Source: CAD feature listing. Evaluate the final solid. Frame: model axes, mm. A direction names the side the tool comes from. Coordinates: 2 decimals unless noted, no trailing zeros. Write each loop counter-clockwise with the first axis right and the second up, starting at its lowest first coordinate (ties: lowest second). Pieces come first, ordered by that corner, then holes. Notation, with made-up numbers: M -27,87 L 13,87 A24 cw 13,125 Z; hole C 85.5,-34 d11. An arc over 180 degrees is marked long. Answer as CSV lines item,"result". Start each with the question number.
1. Section A-A on y = 56.35. Return the cut outline in (x, z) (3 decimals), plus the area to 3 significant figures.
2. Section B-B on z = 1.75. Count the separate pieces of the cut face and the enclosed holes in it, plus the area to 3 significant figures.
3. Section D-D on y = 0. Return the cut outline in (x, z) (3 decimals).
4. Mould query, pull axis Y, two halves, no side actions, for faces 1 (the face through (0, 62.7, 2)), 2 (the face through (-50, 28, 2)), 3 (the face through (-42, 5, 3.175)). Classes: pulls with the +Y half, pulls with the -Y half, needs draft (parallel to the pull), parting line crosses it, or undercut.
5. Contact query for flat-ended pins moving along their axis: pin 1 Ø1.6 at (x, z) = (-58, 2) entering from +Y; pin 2 Ø2 at (x, z) = (48.5, 0.5) entering from -Y; pin 3 Ø3 at (x, z) = (-18.5, 3.5) entering from +Y; pin 4 Ø1.5 at (x, z) = (6, 4) entering from +Y. Output: stop coordinate, or through.
6. Reachability of faces 4 (the face through (-56, 6.35, 2)), 5 (the face through (6.35, 56, 2)), 6 (the face through (1, -40, 2)), 7 (the face through (-6.35, -56, 2)) from +Z, -Z, +X, -X, +Y, -Y: full face, straight path, thin tool, end or side. Return the list, or none.
7. Line query: probe 1 along Y at (x, z) = (43.5, 0.25); probe 2 along Y at (x, z) = (0, 1.9); probe 3 along X at (y, z) = (31, 1.45). Output: solid intervals per line, ascending. Write a range as [from, to].
Autodesk Fusion 360 part; units mm, degrees
sketch "Sketch1" plane through (0, 0, 0) normal (0, 0, 1) x (1, 0, 0) in component "Bracket"
  line L0 (-40, 40) -> (40, 40)
  line L1 (40, 40) -> (40, -40)
  line L2 (40, -40) -> (-40, -40)
  line L3 (-40, -40) -> (-40, 40)
  line L4 (-50, 50) -> (50, 50)
  line L5 (50, 50) -> (50, -50)
  line L6 (50, -50) -> (-50, -50)
  line L7 (-50, -50) -> (-50, 50)
  circle A0 centre (-43.75, 43.75) radius 1
  circle A1 centre (-43.75, -43.75) radius 1
  circle A2 centre (43.75, -43.75) radius 1
  circle A3 centre (43.75, 43.75) radius 1
  line L8 (-6.35, 50) -> (-6.35, 62.7)
  line L9 (-6.35, 62.7) -> (6.35, 62.7)
  line L10 (6.35, 62.7) -> (6.35, 50)
  line L11 (-50, 6.35) -> (-62.7, 6.35)
  line L12 (-62.7, 6.35) -> (-62.7, -6.35)
  line L13 (-62.7, -6.35) -> (-50, -6.35)
  line L14 (-6.35, -50) -> (-6.35, -62.7)
  line L15 (-6.35, -62.7) -> (6.35, -62.7)
  line L16 (6.35, -62.7) -> (6.35, -50)
  line L17 (50, 6.35) -> (62.7, 6.35)
  line L18 (62.7, 6.35) -> (62.7, -6.35)
  line L19 (62.7, -6.35) -> (50, -6.35)
  circle A4 centre (56.35, 0) radius 2.5
  circle A5 centre (0, 56.35) radius 2.5
  circle A6 centre (-56.35, 0) radius 2.5
  circle A7 centre (0, -56.35) radius 2.5
  circle A8 centre (43.75, 43.75) radius 4
  circle A9 centre (-43.75, 43.75) radius 4
  circle A10 centre (-43.75, -43.75) radius 4
  circle A11 centre (43.75, -43.75) radius 4
  dimension "d1" = 80
  dimension "d2" = 80
  dimension "d3" = 100
  dimension "d4" = 100
  dimension "d5" = 40
  dimension "d6" = 50
  dimension "d7" = 40
  dimension "d8" = 50
  dimension "d11" = 2
  dimension "d12" = 2
  dimension "d13" = 2
  dimension "d14" = 2
  dimension "d15" = 87.5
  dimension "d16" = 87.5
  dimension "d17" = 43.75
  dimension "d18" = 43.75
  dimension "d19" = 12.7
  dimension "d20" = 12.7
  dimension "d21" = 6.35
  dimension "d22" = 12.7
  dimension "d23" = 12.7
  dimension "d24" = 6.35
  dimension "d25" = 12.7
  dimension "d26" = 12.7
  dimension "d27" = 6.35
  dimension "d28" = 12.7
  dimension "d29" = 12.7
  dimension "d30" = 6.35
  dimension "d31" = 5
  dimension "d32" = 6.35
  dimension "d33" = 6.35
  dimension "d34" = 5
  dimension "d35" = 6.35
  dimension "d36" = 6.35
  dimension "d37" = 5
  dimension "d38" = 6.35
  dimension "d39" = 6.35
  dimension "d40" = 5
  dimension "d41" = 6.35
  dimension "d42" = 6.35
  dimension "d43" = 8
  dimension "d44" = 8
  dimension "d45" = 8
  dimension "d46" = 8
extrude "Extrude1" add sketch "Sketch1" along normal blind 3.175 contours L4 L5 L6 L7 | L4 L8 L9 L10 | L7 L11 L12 L13 | L5 L17 L18 L19 | L6 L14 L15 L16 in component "Bracket"
extrude "Extrude2" add sketch "Sketch1" along normal blind 5 contours A8 | A9 | A10 | A11 in component "Bracket"
component "Bracket" placed x (1, 0, 0) y (0, 1, 0) z (0, 0, 1) at (0, 0, 0)
equation "d5 = d2 / 2"
equation "d6 = d4 / 2"
equation "d7 = d1 / 2"
equation "d8 = d3 / 2"
equation "d17 = d15 / 2"
equation "d18 = d16 / 2"
Values:
1,outline,"M -6.35,0 L -2.5,0 L -2.5,3.175 L -6.35,3.175 Z; M 2.5,0 L 6.35,0 L 6.35,3.175 L 2.5,3.175 Z"
1,area,"24.4 mm²"
2,separate pieces,"1"
2,enclosed holes,"9"
2,area,"4,150 mm²"
3,outline,"M -62.7,0 L -58.85,0 L -58.85,3.175 L -62.7,3.175 Z; M -53.85,0 L -40,0 L -40,3.175 L -53.85,3.175 Z; M 40,0 L 53.85,0 L 53.85,3.175 L 40,3.175 Z; M 58.85,0 L 62.7,0 L 62.7,3.175 L 58.85,3.175 Z"
4,face 1,"pulls with the +Y half"
4,face 2,"needs draft"
4,face 3,"undercut"
5,pin 1,"y = 6.35"
5,pin 2,"y = -50"
5,pin 3,"y = 50"
5,pin 4,"through"
6,face 4,"+Z, -Z, -X, +Y"
6,face 5,"+Z, -Z, +X, +Y"
6,face 6,"+Z, -Z"
6,face 7,"+Z, -Z, -X, -Y"
7,probe 1,"[-50, -44.72], [-42.78, 42.78], [44.72, 50]"
7,probe 2,"[-62.7, -58.85], [-53.85, -40], [40, 53.85], [58.85, 62.7]"
7,probe 3,"[-50, -40], [40, 50]"
